from build123d import *

# Parameters (mm, degrees)
BASE_FLANGE1_DEPTH           = 115.57
EDGE_FLANGE1_DEPTH           = 115.57
EDGE_FLANGE2_STRIP_CUT_DEPTH = 115.57
EDGE_FLANGE2_DEPTH           = 115.57
EDGE_FLANGE3_DEPTH           = 115.57
SKETCH20_R                   = 7.14375
CUT_EXTRUDE1_DEPTH           = 2.65684


# Sheet-metal steps are written as plain solids
with BuildPart() as part:
    # Sketch1 → Base-Flange1 (new body)
    with BuildSketch(Plane.XY):
        with BuildLine():
            ThreePointArc((-50.8, 170.388379885), (-140.856418383, 108.500273734), (-177.710803869, 5.63118))
            Line((-177.710803869, 5.63118), (-180.366311024, 5.715325918))
            ThreePointArc((-180.366311024, 5.715325918), (-142.961215721, 110.121577824), (-51.559097143, 172.934469105))
            Line((-51.559097143, 172.934469105), (-50.8, 170.388379885))
        make_face()
    extrude(amount=BASE_FLANGE1_DEPTH)

    # Edge-Flange1 section (across the edge) → Edge-Flange1 (add)
    with BuildSketch(Plane(origin=(-49.291175996, 173.610632552, 115.57), x_dir=(-0.9999999996342678, -2.7045604981235094e-05, 0), z_dir=(0, 0, -1))):
        with BuildLine():
            Line((-2.65684, 2.366572064), (-2.65684, 76.2))
            Line((-2.65684, 76.2), (0, 76.2))
            Line((0, 76.2), (0, 2.366572064))
            ThreePointArc((0, 2.366572064), (0.62936233, 0.469112223), (2.267939433, -0.676102109))
            Line((2.267939433, -0.676102109), (1.508911151, -3.222211858))
            ThreePointArc((1.508911151, -3.222211858), (-1.500827273, -1.118682173), (-2.65684, 2.366572064))
        make_face()
    extrude(amount=EDGE_FLANGE1_DEPTH)

    # Edge-Flange2 strip (across the edge) → Edge-Flange2 strip cut (cut)
    with BuildSketch(Plane(origin=(-49.293236871, 249.810632524, 115.57), x_dir=(-0.766027058259036, -0.6428083275868535, 0), z_dir=(0, 0, -1))):
        Polygon((-12.205285278, 10.412383287), (-1.292448625, -2.593029), (0.742808893, -0.885245167), (-10.17002776, 12.12016712), align=None)
    extrude(amount=EDGE_FLANGE2_STRIP_CUT_DEPTH, mode=Mode.SUBTRACT)

    # Edge-Flange2 section (across the edge) → Edge-Flange2 (add)
    with BuildSketch(Plane(origin=(-49.293236871, 249.810632524, 115.57), x_dir=(-0.766027058259036, -0.6428083275868535, 0), z_dir=(0, 0, -1))):
        with BuildLine():
            Line((-2.65684, 1.155605494), (-2.65684, 101.6))
            Line((-2.65684, 101.6), (0, 101.6))
            Line((0, 101.6), (0, 1.155605494))
            ThreePointArc((0, 1.155605494), (0.191475929, 0.069691539), (0.742808893, -0.885245167))
            Line((0.742808893, -0.885245167), (-1.292448625, -2.593029))
            ThreePointArc((-1.292448625, -2.593029), (-2.305137014, -0.839001259), (-2.65684, 1.155605494))
        make_face()
    extrude(amount=EDGE_FLANGE2_DEPTH)

    # Edge-Flange3 section (across the edge) → Edge-Flange3 (add)
    with BuildSketch(Plane(origin=(-180.463740314, 2.640617339, 0), x_dir=(8.626632785422443e-05, 0.9999999962790604, 0), z_dir=(0, 0, 1))):
        with BuildLine():
            Line((-2.65684, 3.076251829), (-2.65684, 57.15))
            Line((-2.65684, 57.15), (0, 57.15))
            Line((0, 57.15), (0, 3.076251829))
            ThreePointArc((0, 3.076251829), (0.894756196, 0.86692768), (3.074716973, -0.097164046))
            Line((3.074716973, -0.097164046), (2.990800136, -2.75267845))
            ThreePointArc((2.990800136, -2.75267845), (-1.013351819, -0.981834768), (-2.65684, 3.076251829))
        make_face()
    extrude(amount=EDGE_FLANGE3_DEPTH)

    # Sketch20 → Cut-Extrude1 (cut)
    with BuildSketch(Plane(origin=(0.000226453, 2.625049375, 0), x_dir=(0.9999999962790604, -8.626632785420363e-05, 0), z_dir=(8.626632785420363e-05, 0.9999999962790604, 0))):
        with Locations(Location((-218.563967439, -31.75, 0), (0, 0, 180))):
            Circle(SKETCH20_R)
        with Locations(Location((-218.563967439, -82.55, 0), (0, 0, 180))):
            Circle(SKETCH20_R)
    extrude(amount=-CUT_EXTRUDE1_DEPTH, mode=Mode.SUBTRACT)


solid = part.part
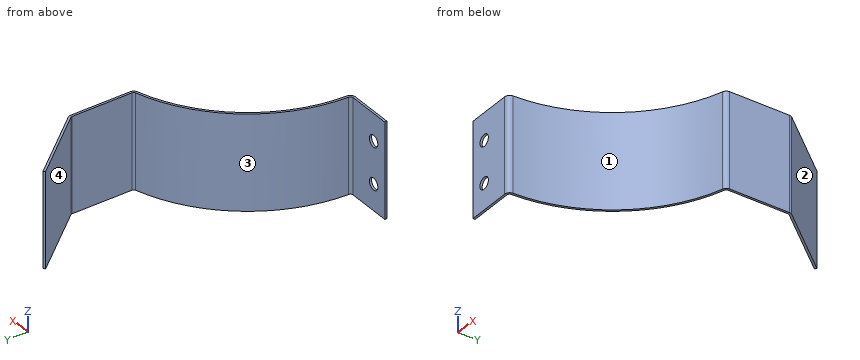
Read the model definition and answer for the solid it produces. Units are mm, in the model's axes. Face numbers are marked on the shaded views. Give positions to 0.01 mm unless a question says otherwise; leave off trailing zeros. Loops run counter-clockwise (first coordinate to the right, second up) from the corner with the lowest first, then second, coordinate; pieces in that order, holes last. Notation, with made-up numbers: (49.5, -29.75) -> (73.5, -29.75) arc R8 ccw to (73.5, -19.75) -> close; hole circle Ø9 at (83.5, 14). An arc over 180 degrees is marked (long way). Use a Markdown table: item, result.
Q1. Find the intervals of material crossed by line 1 along Y through (x, z) = (-82.5, 36); line 2 along Y through (x, z) = (-83, 7); line 3 along X through (y, z) = (226.5, 99), in increasing order.
Solved:
| item | result |
|---|---|
| line 1 | y = 157.5 to 160.49, 289.38 to 293.52 |
| line 2 | y = 157.24 to 160.24, 289.98 to 294.11 |
| line 3 | x = -49.29 to -46.64 |
Q2. Determine the mould class of the marked faces 1, 2, 3 and 4 for opening direction Y: pulls with the +Y half, pulls with the -Y half, needs draft (parallel to the pull), parting line crosses it, or undercut.
Solved:
| item | result |
|---|---|
| face 1 | pulls with the -Y half |
| face 2 | pulls with the +Y half |
| face 3 | undercut |
| face 4 | undercut |
Q3. Section D-D, the plane y = 85.5 is taken. Determine the outline of the cut face in (x, z).
Solved:
| item | result |
|---|---|
| outline | (-158.92, 0) -> (-155.89, 0) -> (-155.89, 115.57) -> (-158.92, 115.57) -> close |
Q4. Section A-A, the plane x = -96.5 is taken. Determine the outline of the cut face in (y, z), then the cut area to 3 significant figures.
Solved:
| item | result |
|---|---|
| outline | (149.33, 0) -> (152.49, 0) -> (152.49, 115.57) -> (149.33, 115.57) -> close; (306.07, 0) -> (310.2, 0) -> (310.2, 115.57) -> (306.07, 115.57) -> close |
| area | 842 mm^2 |
Q5. Each of these flat-tipped pins is pushed along its axis until it touches: pin 1 (22 mm diameter, centred on y = 221.5, z = 58.5, fed in from -X); pin 2 (1 mm diameter, centred on y = 276.5, z = 94.5, fed in from +X); pin 3 (8.5 mm diameter, centred on x = -218.56, z = 82.55, fed in from +Y); pin 4 (12 mm diameter, centred on y = 111, z = 17, fed in from +X). Where does it stop, or does it pass through?
Solved:
| item | result |
|---|---|
| pin 1 | stops at x = -49.29 |
| pin 2 | stops at x = -67.8 |
| pin 3 | passes through |
| pin 4 | stops at x = -133.88 |
Q6. Section B-B, the plane z = 105 is taken. Determine the outline of the cut face in (x, y) (3 decimals), then the cut area to 3 significant figures.
Solved:
| item | result |
|---|---|
| outline | (-237.614, -0.011) -> (-183.54, -0.016) arc R5.832 ccw to (-177.711, 5.631) arc R177.8 cw to (-50.8, 170.388) arc R5.832 ccw to (-46.634, 175.977) -> (-46.636, 248.655) arc R5.832 ccw to (-48.001, 252.404) -> (-112.567, 329.347) -> (-114.603, 327.639) -> (-50.036, 250.696) arc R3.175 cw to (-49.293, 248.655) -> (-49.291, 175.977) arc R3.175 cw to (-51.559, 172.934) arc R180.457 ccw to (-180.366, 5.715) arc R3.175 cw to (-183.54, 2.641) -> (-237.614, 2.646) -> close |
| area | 1,240 mm^2 |
